Part print with two shaded views. Sizes in mm from the minimum x, y, z corner. A direction names the side the tool comes from. Give positions to 0.01 mm unless a question says otherwise; leave off trailing zeros. Order: outer loops, then holes, each group sorted by start corner. A loop starts at its lowest first (then second) coordinate and runs counter-clockwise, first axis right, second up. Notation, with made-up numbers: (50, 59.5) -> (81, 59.5) arc R24 ccw to (81, 92.5) -> close; hole circle Ø6 at (87.25, 69). An arc over 180 degrees is marked (long way). Answer as CSV lines item,"result".
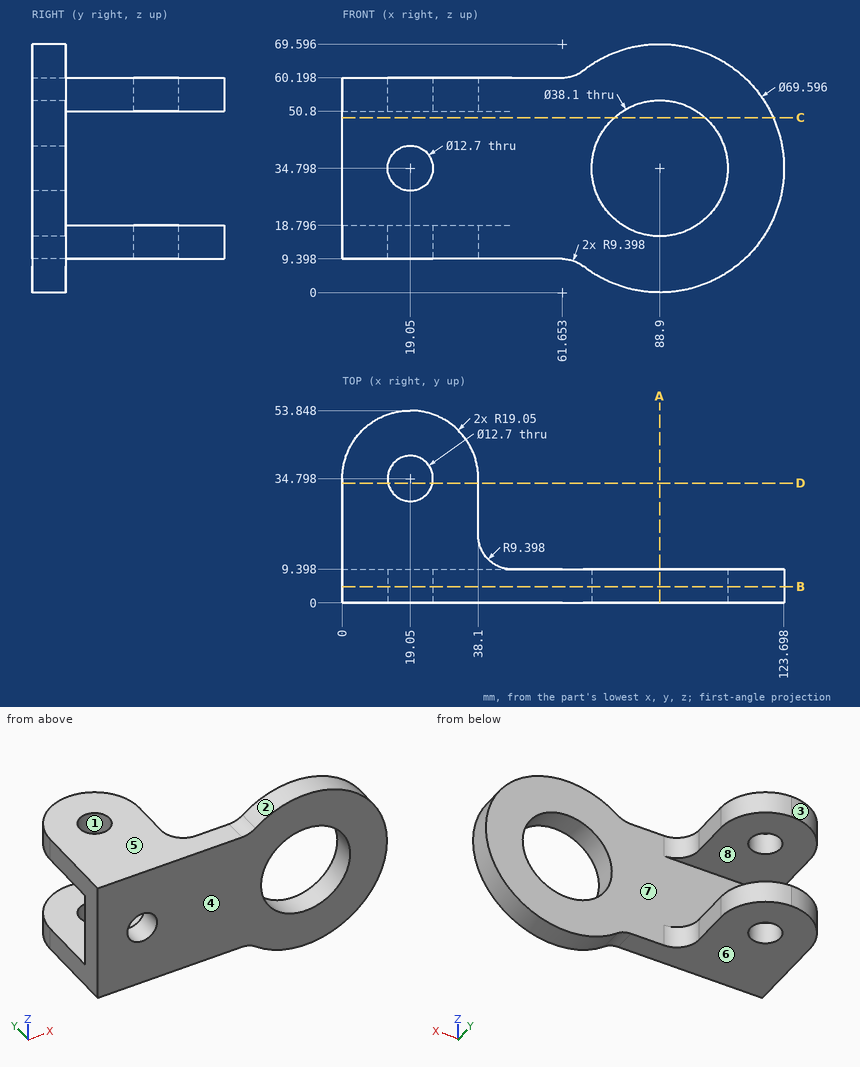
1) Band-saw the part on B-B, the plane y = 4.5. Write the cut outline in (x, z), then the cut area to 3 significant figures.
Data:
outline,"(0, 9.4) -> (61.65, 9.4) arc R9.4 cw to (67.45, 7.4) arc R34.8 ccw (long way) to (67.45, 62.2) arc R9.4 cw to (61.65, 60.2) -> (0, 60.2) -> close; hole circle Ø12.7 at (19.05, 34.8); hole circle Ø38.1 at (88.9, 34.8)"
area,"5,460 mm2"
2) Pull direction Y, two halves, no side cores. Call the marked faces 1, 2, 3 and 4: pulls with the +Y half, pulls with the -Y half, needs draft (parallel to the pull), parting line crosses it, or undercut.
Data:
face 1,"undercut"
face 2,"needs draft"
face 3,"pulls with the +Y half"
face 4,"pulls with the -Y half"
3) Wall check: line 1 along Z through (x, y) = (88, 2); line 2 along Z through (x, y) = (8, 17); line 3 along Y through (x, z) = (19, 53). Give the ranges that are in metal, low to high. Write a range as [from, to].
Data:
line 1,"z = [0.01, 15.77], [53.83, 69.58]"
line 2,"z = [9.4, 18.8], [50.8, 60.2]"
line 3,"y = [0, 28.45], [41.15, 53.85]"
4) Band-saw the part on C-C, the plane z = 49. Write the cut outline in (x, y).
Data:
outline,"(0, 0) -> (76.2, 0) -> (76.2, 9.4) -> (0, 9.4) -> close; (101.6, 0) -> (120.67, 0) -> (120.67, 9.4) -> (101.6, 9.4) -> close"
5) Band-saw the part on D-D, the plane y = 33.5. Write the cut outline in (x, z).
Data:
outline,"(0, 9.4) -> (12.83, 9.4) -> (12.83, 18.8) -> (0, 18.8) -> close; (0, 50.8) -> (12.83, 50.8) -> (12.83, 60.2) -> (0, 60.2) -> close; (25.27, 9.4) -> (38.1, 9.4) -> (38.1, 18.8) -> (25.27, 18.8) -> close; (25.27, 50.8) -> (38.1, 50.8) -> (38.1, 60.2) -> (25.27, 60.2) -> close"
6) Band-saw the part on A-A, the plane x = 88.9. Write the cut outline in (y, z), then the cut area to 3 significant figures.
Data:
outline,"(0, 0) -> (9.4, 0) -> (9.4, 15.75) -> (0, 15.75) -> close; (0, 53.85) -> (9.4, 53.85) -> (9.4, 69.6) -> (0, 69.6) -> close"
area,"296 mm2"
7) Pin check, flat tips, straight feed: P1, Ø1.5, axis at x = 64, y = 9.5, coming from the +Z side; P2, Ø10, axis at x = 19.05, y = 34.798, coming from the +Z side; P3, Ø7.5, axis at y = 27.5, z = 16, coming from the +X side. Stop position of each tip, or through.
Data:
P1,"stops at z = 60.72"
P2,"passes through"
P3,"stops at x = 38.1"
8) Which spindle directions (+Z, -Z, +X, -X, +Y, -Y) get a long thin tool onto all of the face, cutting with end or side? Do the marked faces 5, 6, 7 and 8. Say none if no direction does.
Data:
face 5,"+Z, -X, +Y, -Y"
face 6,"-Z, -X, +Y, -Y"
face 7,"+X, +Y"
face 8,"+X, -X, +Y"
